from build123d import *

# Parameters (mm, degrees)
SKETCH_W             = 31
SKETCH_H             = 31.5
PAD_DEPTH            = 12
PAD_DEPTH_BACK       = 10
POCKET_DEPTH         = 21
SKETCH002_W          = 26.4
SKETCH002_H          = 22.8
SKETCH002_W_2        = 18
SKETCH002_H_2        = 6
POCKET001_DEPTH      = 19
SKETCH003_W          = 9
SKETCH003_H          = 5
POCKET002_DEPTH      = 4.5
POCKET002_DEPTH_BACK = 15
POCKET003_DEPTH      = 6.501
SKETCH005_W          = 16
SKETCH005_H          = 3.6
POCKET004_DEPTH      = 1
SKETCH006_R          = 2
POCKET005_DEPTH      = 25.001
HOLE_D               = 2.8
HOLE_DEPTH           = 14
HOLE_CBORE_D         = 4.5
HOLE_CBORE_DEPTH     = 5
HOLE_TIPS_R          = 1.4
SKETCH008_R          = 2.5
POCKET006_DEPTH      = 15.501


with BuildPart() as part:
    # Sketch → Pad (new body, two sides)
    with BuildSketch(Plane.XY) as pad_sk:
        with Locations((0, 9.25)):
            Rectangle(SKETCH_W, SKETCH_H)
    extrude(amount=PAD_DEPTH)
    extrude(pad_sk.sketch, amount=-PAD_DEPTH_BACK)

    # Sketch001 → Pocket (cut)
    with BuildSketch(Plane.XY.offset(12)):
        Polygon((-7.9, -2.85), (-7.9, -1), (-10.5, -1), (-10.5, -2.85), (-13.2, -2.85), (-13.2, -0.65), (-13.7, -0.65), (-13.7, 0.65), (-13.2, 0.65), (-13.2, 4.45), (13.2, 4.45), (13.2, 0.65), (13.7, 0.65), (13.7, -0.65), (13.2, -0.65), (13.2, -2.85), (10.5, -2.85), (10.5, -1), (7.9, -1), (7.9, -2.85), align=None)
    extrude(amount=-POCKET_DEPTH, mode=Mode.SUBTRACT)

    # Sketch002 → Pocket001 (cut)
    with BuildSketch(Plane.XY.offset(12)):
        with Locations((0, 12.05)):
            Rectangle(SKETCH002_W, SKETCH002_H)
        with Locations((0, 7.45)):
            Rectangle(SKETCH002_W_2, SKETCH002_H_2, mode=Mode.SUBTRACT)
    extrude(amount=-POCKET001_DEPTH, mode=Mode.SUBTRACT)

    # Sketch003 → Pocket002 (cut, two sides)
    with BuildSketch(Plane.XY) as pocket002_sk:
        with Locations((0, -2.5)):
            Rectangle(SKETCH003_W, SKETCH003_H)
    extrude(amount=-POCKET002_DEPTH, mode=Mode.SUBTRACT)
    extrude(pocket002_sk.sketch, amount=POCKET002_DEPTH_BACK, mode=Mode.SUBTRACT)

    # Sketch004 → Pocket003 (cut, through all)
    with BuildSketch(Plane.XZ):
        with BuildLine():
            ThreePointArc((-4, 0), (0, -4), (4, 0))
            Line((5.2, 0), (4, 0))
            Line((7.9, 12), (5.2, 0))
            Line((-7.9, 12), (7.9, 12))
            Line((-5.2, 0), (-7.9, 12))
            Line((-4, 0), (-5.2, 0))
        make_face()
    extrude(amount=POCKET003_DEPTH, mode=Mode.SUBTRACT)

    # Sketch005 → Pocket004 (cut)
    with BuildSketch(Plane.XY.offset(-10)):
        with Locations((0, -1.8)):
            Rectangle(SKETCH005_W, SKETCH005_H)
    extrude(amount=POCKET004_DEPTH, mode=Mode.SUBTRACT)

    # Sketch006 → Pocket005 (cut, through all)
    with BuildSketch(Plane.XZ):
        with Locations((9.5, -5)):
            Circle(SKETCH006_R)
    extrude(amount=-POCKET005_DEPTH, mode=Mode.SUBTRACT)

    # Hole
    with Locations(Plane.XY.offset(12)):
        with Locations((0, 7.5)):
            CounterBoreHole(HOLE_D / 2, HOLE_CBORE_D / 2, HOLE_CBORE_DEPTH, depth=HOLE_DEPTH)

    # Hole tips → Hole tip 1 section 0
    with BuildSketch(Plane.XY.offset(-2), mode=Mode.PRIVATE) as hole_tip_1_s0:
        with Locations((0, 7.5)):
            Circle(HOLE_TIPS_R)
    loft([hole_tip_1_s0.sketch, Vertex(0, 7.5, -2.841205)], mode=Mode.SUBTRACT)

    # Sketch008 → Pocket006 (cut, through all)
    with BuildSketch(Plane.YZ):
        with Locations((15.858465, 6.985507)):
            Circle(SKETCH008_R)
    extrude(amount=POCKET006_DEPTH, mode=Mode.SUBTRACT)


solid = part.part
Source: CAD feature listing. Evaluate the final solid. Frame: model axes, mm. A direction names the side the tool comes from. Coordinates: 2 decimals unless noted, no trailing zeros. Loops run counter-clockwise (first coordinate to the right, second up) from the corner with the lowest first, then second, coordinate; pieces in that order, holes last. Notation, with made-up numbers: (89, 15.25) - (104, 15.25) arc R18 ccw to (104, 34.25) - close; hole circle Ø1 at (62.5, -38.5). An arc over 180 degrees is marked (long way). One line per item, written item: value. Start each with the question number.
1. Section C-C (y = 19.5). Return the cut outline in (x, z), and give its area (3 significant figures).
2. Mould query, pull axis X, two halves, no side actions, for faces 1 (the flat face through (6.57, -4.65, 6.08)), 2 (the flat face through (15.5, 9, 1)), 3 (the flat face through (-4, -6.5, -4)). Classes: pulls with the +X half, pulls with the -X half, needs draft (parallel to the pull), parting line crosses it, or undercut.
3. Set-up query: faces 4 (the flat face through (0, 25, 1)), 5 (the cylindrical face through (0, -6, -4)), 6 (the flat face through (-10.5, -2, 2)), 7 (the flat face through (0, -3.2, -9)), 8 (the flat face through (0, -2.85, -5)). Return all of +Z, -Z, +X, -X, +Y, -Y with unobstructed straight access to the full face (end or side cutting, diameter ignored); none if empty.
4. Section B-B (x = 3). Return the cut outline in (y, z), and give its area (3 significant figures).
5. Section D-D (z = -1.5). State how many separate pieces and enclosed holes the cut face has, and give its area (3 significant figures).
6. Ray query, L1, parallel to Y at x = 0, z = 10.2; L2, parallel to Y at x = 0, z = -4.25; L3, parallel to X at y = 22, z = 9. Return the intervals inside material, ascending.
Verdict:
1. outline: (-15.5, -10) - (15.5, -10) - (15.5, 12) - (13.2, 12) - (13.2, -7) - (-13.2, -7) - (-13.2, 12) - (-15.5, 12) - close
1. area: 180 mm2
2. face 1: undercut
2. face 2: pulls with the +X half
2. face 3: needs draft
3. face 4: +Z, -Z, +X, -X, +Y
3. face 5: +Z, -Y
3. face 6: +Z
3. face 7: -Z
3. face 8: +Z, -Z
4. outline: (-6.5, -10) - (-3.6, -10) - (-3.6, -9) - (-2.85, -9) - (-2.85, -4.5) - (-5, -4.5) - (-5, -2.65) - (-6.5, -2.65) - close; (0, -10) - (25, -10) - (25, 12) - (23.45, 12) - (23.45, -7) - (10.45, -7) - (10.45, 12) - (4.45, 12) - (4.45, -9) - (0, -9) - close
4. area: 232 mm2
5. separate pieces: 2
5. enclosed holes: 1
5. area: 362 mm2
6. L1: y = 4.45 to 5.25, 9.75 to 10.45, 23.45 to 25
6. L2: y = -6.5 to -5, 4.45 to 10.45, 23.45 to 25
6. L3: x = -15.5 to -13.2, 13.2 to 15.5
